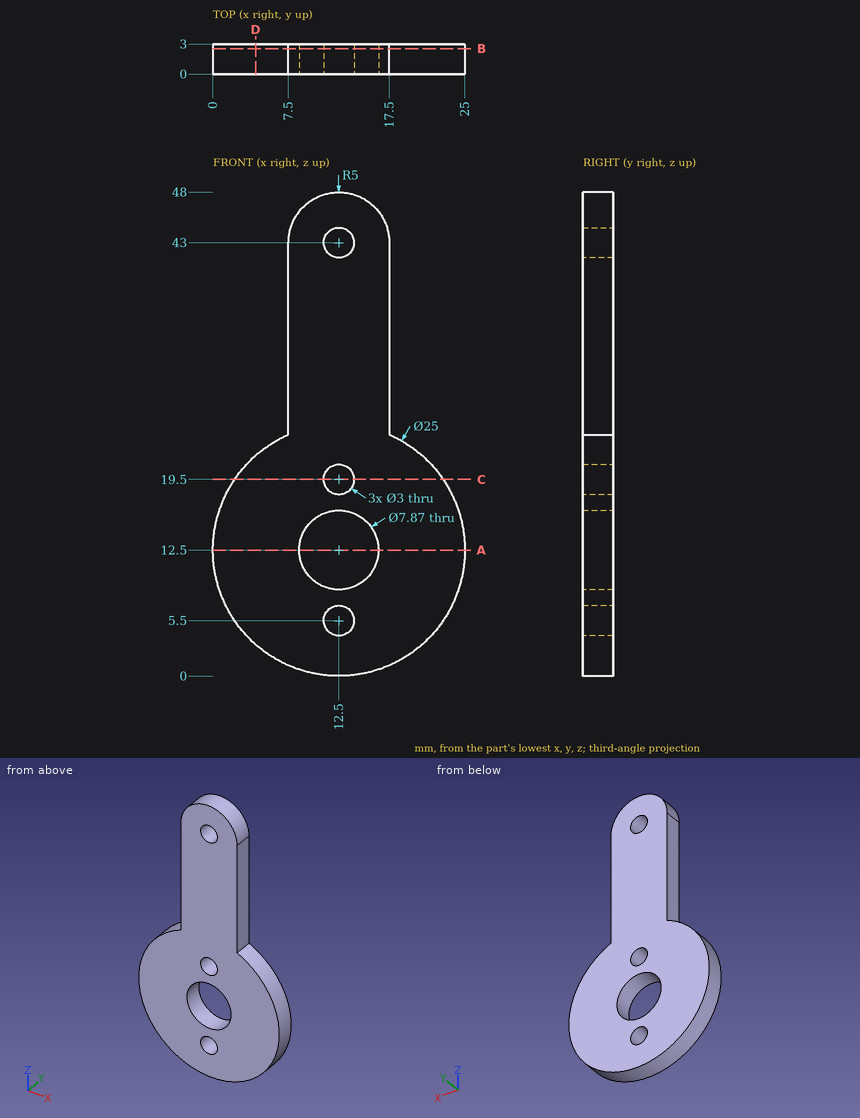
Geometry check sheet. Reference: drawing and pictorial views, mm from the part's lowest x, y, z. Round coordinates to 2 decimals unless told otherwise and drop trailing zeros. Loops run counter-clockwise (first coordinate to the right, second up) from the corner with the lowest first, then second, coordinate; pieces in that order, holes last. Notation, with made-up numbers: M -18,64 L 35,64 A14 ccw 35,78 Z; hole C 65,38.5 d6. An arc over 180 degrees is marked long. One line per item, written item: value.
(1) Sectioned sample at A-A, the plane z = 12.5. Record the cut outline in (x, y) (3 decimals), then the cut area to 3 significant figures.
Computed values:
outline: M 0,0 L 8.565,0 L 8.565,3 L 0,3 Z; M 16.435,0 L 25,0 L 25,3 L 16.435,3 Z
area: 51.4 mm^2
(2) Sectioned sample at B-B, the plane y = 2.55. Record the cut outline in (x, z) (3 decimals).
Computed values:
outline: M 7.5,23.956 A12.5 ccw long 17.5,23.956 L 17.5,43 A5 ccw 7.5,43 Z; hole C 12.5,12.5 d7.87; hole C 12.5,5.5 d3; hole C 12.5,19.5 d3; hole C 12.5,43 d3
(3) Sectioned sample at C-C, the plane z = 19.5. Record the cut outline in (x, y).
Computed values:
outline: M 2.14,0 L 11,0 L 11,3 L 2.14,3 Z; M 14,0 L 22.86,0 L 22.86,3 L 14,3 Z
(4) Depth check by flat-ended pin: pin 1 Ø1.5 at (y, z) = (2, 37.5) entering from -X; pin 2 Ø4 at (x, z) = (12.5, 43) entering from -Y; pin 3 Ø1 at (x, y) = (21.5, 0.5) entering from +Z; pin 4 Ø1 at (x, y) = (8, 1) entering from -Z. Enter the tip coordinate at first touch or a pass-through.
Computed values:
pin 1: stops at x = 7.5
pin 2: stops at y = 0
pin 3: stops at z = 21.67
pin 4: stops at z = 0.66
(5) Thickness scan on line 1 (Z direction, x = 12.5, y = 0.85) (3 decimals); line 2 (X direction, y = 2.2, z = 43); line 3 (X direction, y = 2.4, z = 12.5) (3 decimals). Record the ranges inside material, lowest first.
Computed values:
line 1: z = 0 to 4, 7 to 8.565, 16.435 to 18, 21 to 41.5, 44.5 to 48
line 2: x = 7.5 to 11, 14 to 17.5
line 3: x = 0 to 8.565, 16.435 to 25
(6) Sectioned sample at D-D, the plane x = 4.25. Record the cut outline in (y, z), then the cut area to 3 significant figures.
Computed values:
outline: M 0,3.11 L 3,3.11 L 3,21.89 L 0,21.89 Z
area: 56.3 mm^2
